```python
from build123d import *

# Parameters (mm, degrees)
SKETCH007_W     = 18
SKETCH007_H     = 18
PAD007_DEPTH    = 20
THICKNESS002_T  = -1.2
SKETCH008_R     = 3.25
POCKET002_DEPTH = 5
SKETCH009_W     = 3.3
SKETCH009_H     = 15.6
PAD008_DEPTH    = 18.8
SKETCH010_R     = 1.45
POCKET003_DEPTH = 18.001


with BuildPart() as part:
    # Sketch007 → Pad007 (new body)
    with BuildSketch(Plane.XY):
        with Locations((9, 9)):
            Rectangle(SKETCH007_W, SKETCH007_H)
    extrude(amount=PAD007_DEPTH)

    # Thickness002
    thickness002_openings = [part.faces().sort_by_distance(p)[0] for p in [
        (9, 9, 0),
    ]]
    offset(amount=THICKNESS002_T, openings=thickness002_openings, kind=Kind.INTERSECTION)

    # Sketch008 (on Face5 of Thickness002) → Pocket002 (cut)
    with BuildSketch(Plane.XY.offset(20)):
        with Locations((9, 9)):
            Circle(SKETCH008_R)
    extrude(amount=-POCKET002_DEPTH, mode=Mode.SUBTRACT)

    # Sketch009 (on Face4 of Pocket002) → Pad008 (join)
    with BuildSketch(Plane(origin=(0, 0, 0), x_dir=(1, 0, 0), z_dir=(0, 0, -1))):
        with Locations((2.85, -9)):
            Rectangle(SKETCH009_W, SKETCH009_H)
        with Locations((15.15, -9)):
            Rectangle(SKETCH009_W, SKETCH009_H)
    extrude(amount=-PAD008_DEPTH)

    # Sketch010 (on Face6 of Pad008) → Pocket003 (cut, through all)
    with BuildSketch(Plane(origin=(0, 18, 0), x_dir=(-1, 0, 0), z_dir=(0, 1, 0))):
        with Locations((-15.8, 10)):
            Circle(SKETCH010_R)
        with Locations((-2.2, 10)):
            Circle(SKETCH010_R)
    extrude(amount=-POCKET003_DEPTH, mode=Mode.SUBTRACT)


with BuildPart() as part_1:
    # Body003 placement: moved
    add(part.part.moved(Location((-75, 0, 0))))


solid = part_1.part
```
Geometry: final body of the model. Coordinates: model frame, mm. A direction names the side the tool comes from. Round coordinates to 2 decimals unless told otherwise and drop trailing zeros. Loops run counter-clockwise (first coordinate to the right, second up) from the corner with the lowest first, then second, coordinate; pieces in that order, holes last. Notation, with made-up numbers: (-25, -17) -> (-15, -17) arc R14 ccw to (-15, -4) -> close; hole circle Ø11 at (-17, 43). An arc over 180 degrees is marked (long way). Use one line per item in the form item = value.
Item 1: Cut plane C-C on x = -72.75. Output: boundary loops of the cut face in (y, z), then the cut area to 3 significant figures.
Evaluation:
outline = (0, 0) -> (18, 0) -> (18, 8.55) -> (0, 8.55) -> close; (0, 11.45) -> (18, 11.45) -> (18, 20) -> (0, 20) -> close
area = 308 mm2
Item 2: Cut plane D-D on y = 4.25. Output: boundary loops of the cut face in (x, z), then the cut area to 3 significant figures.
Evaluation:
outline = (-75, 0) -> (-70.5, 0) -> (-70.5, 18.8) -> (-61.5, 18.8) -> (-61.5, 0) -> (-57, 0) -> (-57, 20) -> (-75, 20) -> close; hole circle Ø2.9 at (-72.8, 10); hole circle Ø2.9 at (-59.2, 10)
area = 178 mm2
Item 3: Draft query along Y for faces 3 (the flat face through (-61.5, 9, 9)), 4 (the flat face through (-70, 9, 20)), 5 (the flat face through (-66, 0, 10)), 6 (the flat face through (-66, 18, 10)). Return one class per face: released by +Y, released by -Y, zero draft, split by the parting line, or undercut.
Evaluation:
face_3 = undercut
face_4 = zero draft
face_5 = released by -Y
face_6 = released by +Y
Item 4: Access query for faces 1 (the cylindrical face through (-71.35, 9.13, 10.06)), 2 (the flat face through (-69, 7, 18.8)). Directions: +Z, -Z, +X, -X, +Y, -Y. A direction counts if a zero-diameter tool reaches every point of the face in a straight line with its end or side. Return the directions, or none.
Evaluation:
face_1 = +Y, -Y
face_2 = -Z
Item 5: Cut plane B-B on z = 10. Output: boundary loops of the cut face in (x, y), then the cut area to 3 significant figures.
Evaluation:
outline = (-75, 0) -> (-74.25, 0) -> (-74.25, 18) -> (-75, 18) -> close; (-71.35, 0) -> (-60.65, 0) -> (-60.65, 18) -> (-71.35, 18) -> close; (-57.75, 0) -> (-57, 0) -> (-57, 18) -> (-57.75, 18) -> close; hole (-70.5, 1.2) -> (-61.5, 1.2) -> (-61.5, 16.8) -> (-70.5, 16.8) -> close
area = 79.2 mm2
Item 6: Material intervals for probe 1 along Y at (x, z) = (-63.5, 18); probe 2 along X at (y, z) = (12.5, 6); probe 3 along X at (y, z) = (1, 9), sorted ascending.
Evaluation:
probe_1 = 0 to 1.2, 16.8 to 18
probe_2 = -75 to -70.5, -61.5 to -57
probe_3 = -75 to -73.85, -71.75 to -60.25, -58.15 to -57
Item 7: Contact query for flat-ended pins moving along their axis: pin 1 Ø4 at (x, z) = (-68.5, 9) entering from -Y; pin 2 Ø2.5 at (x, z) = (-72.8, 10) entering from -Y; pin 3 Ø2.5 at (x, y) = (-65.5, 11) entering from -Z. Output: stop coordinate, or through.
Evaluation:
pin_1 = 0
pin_2 = through
pin_3 = 18.8
Item 8: Cut plane A-A on y = 9. Output: boundary loops of the cut face in (x, z).
Evaluation:
outline = (-75, 0) -> (-70.5, 0) -> (-70.5, 18.8) -> (-69.25, 18.8) -> (-69.25, 20) -> (-75, 20) -> close; (-62.75, 18.8) -> (-61.5, 18.8) -> (-61.5, 0) -> (-57, 0) -> (-57, 20) -> (-62.75, 20) -> close; hole circle Ø2.9 at (-72.8, 10); hole circle Ø2.9 at (-59.2, 10)
